Source: three-view drawing plus pictorial views. Frame: mm from the lowest corner of the part. A direction names the side the tool comes from. Give positions to 0.01 mm unless a question says otherwise; leave off trailing zeros. Loops run counter-clockwise (first coordinate to the right, second up) from the corner with the lowest first, then second, coordinate; pieces in that order, holes last.
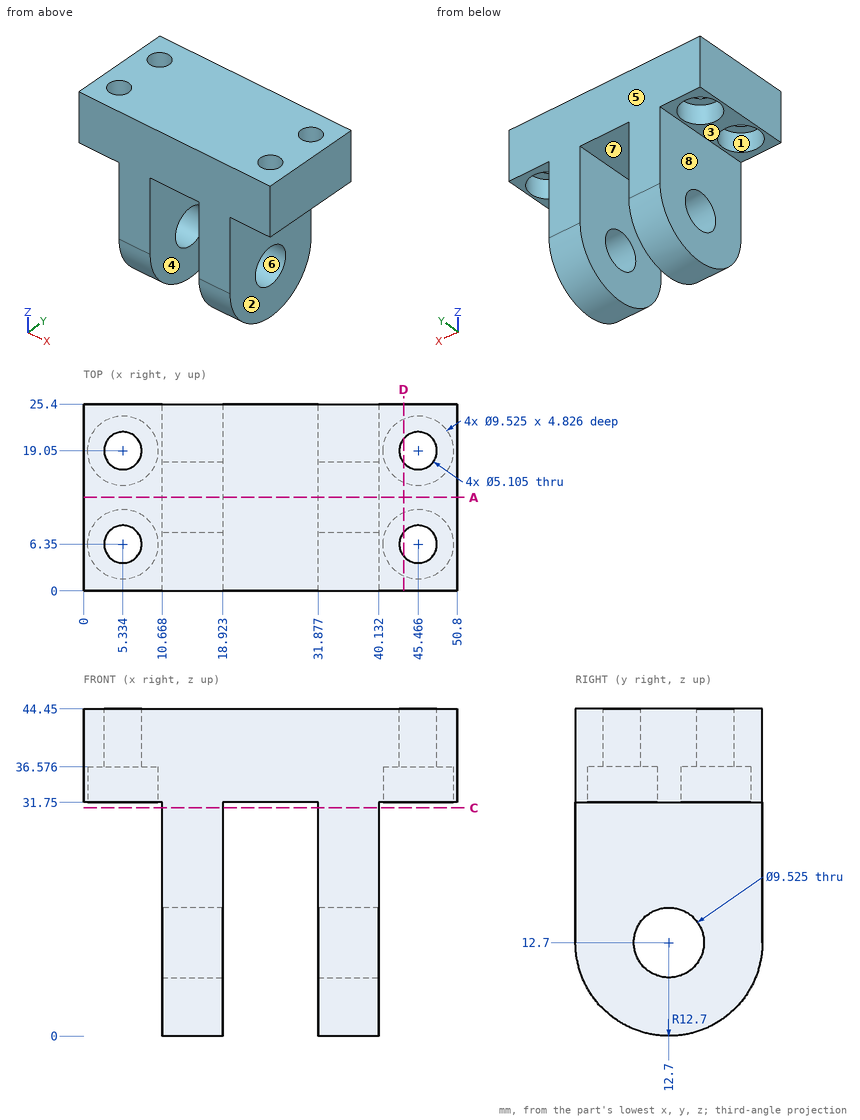
1) Pull-direction query (Z, two-part tool) for the marked faces 6, 7 and 8; classes: released by +Z, released by -Z, zero draft, split by the parting line, or undercut.
Checks:
face 6: undercut
face 7: released by -Z
face 8: zero draft
2) Cut plane D-D (x = 43.5). Return loops of the section in (y, z).
Checks:
outline: (0, 31.75) - (2.01, 31.75) - (2.01, 36.58) - (4.72, 36.58) - (4.72, 44.45) - (0, 44.45) - close; (7.98, 36.58) - (10.69, 36.58) - (10.69, 31.75) - (14.71, 31.75) - (14.71, 36.58) - (17.42, 36.58) - (17.42, 44.45) - (7.98, 44.45) - close; (20.68, 36.58) - (23.39, 36.58) - (23.39, 31.75) - (25.4, 31.75) - (25.4, 44.45) - (20.68, 44.45) - close
3) Cut plane A-A (y = 12.7). Return loops of the section in (x, z), and give its area (3 significant figures).
Checks:
outline: (0, 31.75) - (10.67, 31.75) - (10.67, 17.46) - (18.92, 17.46) - (18.92, 31.75) - (31.88, 31.75) - (31.88, 17.46) - (40.13, 17.46) - (40.13, 31.75) - (50.8, 31.75) - (50.8, 44.45) - (0, 44.45) - close; (10.67, 0) - (18.92, 0) - (18.92, 7.94) - (10.67, 7.94) - close; (31.88, 0) - (40.13, 0) - (40.13, 7.94) - (31.88, 7.94) - close
area: 1,010 mm2
4) Reachability of the marked faces 1, 2, 3, 4 and 5 from +Z, -Z, +X, -X, +Y, -Y: full face, straight path, thin tool, end or side. Return the list, or none.
Checks:
face 1: -Z
face 2: -Z, +X, +Y, -Y
face 3: -Z, -X, +Y, -Y
face 4: -Z, +Y, -Y
face 5: +Z, -Z, +X, -X, +Y
5) Ray query, probe 1 along Z at (x, y) = (13.5, 12.7); probe 2 along X at (y, z) = (23.5, 11); probe 3 along Y at (x, z) = (44.5, 40.5). Return the intervals inside material, ascending.
Checks:
probe 1: z = 0 to 7.94, 17.46 to 44.45
probe 2: x = 10.67 to 18.92, 31.88 to 40.13
probe 3: y = 0 to 3.99, 8.71 to 16.69, 21.41 to 25.4
6) Cut plane C-C (z = 31). Return loops of the section in (x, y), and give its area (3 significant figures).
Checks:
outline: (10.67, 0) - (18.92, 0) - (18.92, 25.4) - (10.67, 25.4) - close; (31.88, 0) - (40.13, 0) - (40.13, 25.4) - (31.88, 25.4) - close
area: 419 mm2
7) Contact query for flat-ended pins moving along their axis: P1, Ø12.5, axis at x = 5.334, y = 19.05, coming from the +Z side; P2, Ø12.5, axis at y = 7, z = 19.5, coming from the +X side; P3, Ø6, axis at y = 7, z = 15.5, coming from the -X side; P4, Ø10.5, axis at x = 27.5, y = 8, coming from the -Z side. Output: stop coordinate, or through.
Checks:
P1: stops at z = 44.45
P2: stops at x = 40.13
P3: stops at x = 10.67
P4: stops at z = 0.13
